```python
from build123d import *

# Parameters (mm, degrees)
BOSS_EXTRUDE1_DEPTH = 2.5
SKETCH2_R           = 1.5
CUT_EXTRUDE1_DEPTH  = 151.793609014
SKETCH3_R           = 1.75
CUT_EXTRUDE2_DEPTH  = 151.793609014


with BuildPart() as part:
    # Sketch1 → Boss-Extrude1 (new, symmetric)
    with BuildSketch(Plane(origin=(0, 0, 0), x_dir=(1, 0, 0), z_dir=(0, 1, 0))):
        Polygon((0, 18.32), (-93.530963622, 61.934204612), (-97.099562891, 68.014303234), (-117.038334206, 77.311904992), (-118.728807253, 73.686673844), (-122.354038401, 75.377146891), (-125.861769973, 67.854792259), (-129.369941895, 60.33264298), (-125.744809712, 58.641957717), (-127.435494976, 55.016825534), (-107.497267972, 45.718056586), (-100.545722072, 46.892156069), (-7.017311764, 3.272476275), (0, 0), (7.017311764, 3.272476275), (100.545722072, 46.892156069), (107.497267972, 45.718056586), (127.435494976, 55.016825534), (125.744809712, 58.641957717), (129.369941895, 60.33264298), (125.861769973, 67.854792259), (122.354038401, 75.377146891), (118.728807253, 73.686673844), (117.038334206, 77.311904992), (97.099562891, 68.014303234), (93.530963622, 61.934204612), align=None)
    extrude(amount=BOSS_EXTRUDE1_DEPTH, both=True)

    # Sketch2 → Cut-Extrude1 (cut, through all)
    with BuildSketch(Plane(origin=(0, 2.5, 0), x_dir=(1, 0, 0), z_dir=(0, 1, 0))):
        with Locations(Location((-11, 14.291347512, 0), (0, 0, 270))):
            Circle(SKETCH2_R)
        with Locations(Location((11, 14.291347512, 0), (0, 0, 270))):
            Circle(SKETCH2_R)
        with Locations(Location((-27, 21.752270043, 0), (0, 0, 270))):
            Circle(SKETCH2_R)
        with Locations(Location((27, 21.752270043, 0), (0, 0, 90))):
            Circle(SKETCH2_R)
    extrude(amount=-CUT_EXTRUDE1_DEPTH, mode=Mode.SUBTRACT)

    # Sketch3 → Cut-Extrude2 (cut, through all)
    with BuildSketch(Plane(origin=(0, 2.5, 0), x_dir=(1, 0, 0), z_dir=(0, 1, 0))):
        with Locations(Location((-114.001493892, 68.562429851, 0), (0, 0, 270))):
            Circle(SKETCH3_R)
        with Locations(Location((-118.780213306, 58.314432997, 0), (0, 0, 270))):
            Circle(SKETCH3_R)
        with Locations(Location((-103.742089693, 63.778391104, 0), (0, 0, 270))):
            Circle(SKETCH3_R)
        with Locations(Location((-108.521689093, 53.530073465, 0), (0, 0, 270))):
            Circle(SKETCH3_R)
        with Locations(Location((103.742089693, 63.778391104, 0), (0, 0, 90))):
            Circle(SKETCH3_R)
        with Locations(Location((108.521689093, 53.530073465, 0), (0, 0, 90))):
            Circle(SKETCH3_R)
        with Locations(Location((118.780213306, 58.314432997, 0), (0, 0, 90))):
            Circle(SKETCH3_R)
        with Locations(Location((114.001493892, 68.562429851, 0), (0, 0, 90))):
            Circle(SKETCH3_R)
    extrude(amount=-CUT_EXTRUDE2_DEPTH, mode=Mode.SUBTRACT)


solid = part.part
```
Geometry check sheet. Reference: the model listing, model coordinates, mm. A direction names the side the tool comes from. Give positions to 0.01 mm unless a question says otherwise; leave off trailing zeros. Order: outer loops, then holes, each group sorted by start corner. A loop starts at its lowest first (then second) coordinate and runs counter-clockwise, first axis right, second up.
1. Section check C-C, the plane y = 0.95. Give the number of separate pieces and of enclosed holes in the cut face, and give its area (3 significant figures).
2. Thickness scan on L1, parallel to X at y = -0.25, z = -55; L2, parallel to X at y = 1.7, z = -50; L3, parallel to X at y = 0.65, z = -48.5. Record the ranges inside material, lowest first.
3. Release check for a two-part mould opening along X. For faces 1 (the face through (-106.93, 0.04, -72.6)), 2 (the face through (117.327, 0.035, -50.302)), 3 (the face through (-10, 2.5, -22)) record: pulls with the +X half, pulls with the -X half, needs draft (parallel to the pull), parting line crosses it, or undercut.
4. Section check B-B, the plane x = -18.5. Enter the section's corners in (y, z).
5. Section check A-A, the plane z = -42. Enter the section's corners in (x, y).
6. Gauge pin test, flat ends, axial feed: pin 1 Ø2 at (x, z) = (108.52, -53.53) entering from +Y; pin 2 Ø2 at (y, z) = (-1.5, -39.5) entering from +X; pin 3 Ø1.5 at (y, z) = (0, -49.5) entering from -X. Record the tip position at first contact, or that the pin passes through.
7. Section check D-D, the plane x = 81. Enter the section's corners in (y, z), and give its area (3 significant figures).
8. Access from +Z, -Z, +X, -X, +Y, -Y to the whole of each face (thin tool, end or side, straight path). Record for faces 4 (the face through (-104.07, 0.035, -46.297)), 5 (the face through (107.21, 0.04, -72.73)), 6 (the face through (-117.606, 0.035, -50.433)).
Values follow:
1. separate pieces: 1
1. enclosed holes: 12
1. area: 4,900 mm2
2. L1: x = -127.4 to -109.47, -107.57 to -78.66, 78.66 to 107.57, 109.47 to 127.4
2. L2: x = -116.68 to -67.94, 67.94 to 116.68
2. L3: x = -113.46 to -64.72, 64.72 to 113.46
3. face 1: undercut
3. face 2: pulls with the +X half
3. face 3: needs draft
4. outline: (-2.5, -26.95) - (2.5, -26.95) - (2.5, -8.63) - (-2.5, -8.63) - close
5. outline: (-90.06, -2.5) - (-50.78, -2.5) - (-50.78, 2.5) - (-90.06, 2.5) - close; (50.78, -2.5) - (90.06, -2.5) - (90.06, 2.5) - (50.78, 2.5) - close
6. pin 1: passes through
6. pin 2: stops at x = 86.84
6. pin 3: stops at x = -117.21
7. outline: (-2.5, -56.09) - (2.5, -56.09) - (2.5, -37.78) - (-2.5, -37.78) - close
7. area: 91.6 mm2
8. face 4: +Z, +Y, -Y
8. face 5: -Z, +Y, -Y
8. face 6: +Z, -X, +Y, -Y
